```python
from build123d import *

# Parameters (mm, degrees)
F0_W     = 158.75
F0_H     = 6.35
F0_W_2   = 6.35
F0_H_2   = 95.25
F1_DEPTH = 19.05
F2_R     = 2.032
F3_DEPTH = 15.24
F4_R     = 2.032
F5_DEPTH = 25.4


with BuildPart() as f1:
    # F0 (on Top) → F1 (new body)
    with BuildSketch(Plane.XY):
        with Locations((-7.746776, 11.7905)):
            Rectangle(F0_W, F0_H)
        with Locations((74.803224, 11.7905)):
            Rectangle(F0_W_2, F0_H)
        with Locations((74.803224, -39.0095)):
            Rectangle(F0_W_2, F0_H_2)
    extrude(amount=F1_DEPTH)

    # F2 (on face) → F3 (cut)
    with BuildSketch(Plane.XZ.offset(86.6345)):
        with Locations((74.803224, 15.875)):
            Circle(F2_R)
        with Locations((74.803224, 3.175)):
            Circle(F2_R)
    extrude(amount=-F3_DEPTH, mode=Mode.SUBTRACT)

    # F4 (on face) → F5 (cut)
    with BuildSketch(Plane(origin=(0, 14.9655, 0), x_dir=(-1, 0, 0), z_dir=(0, 1, 0))):
        with Locations((83.946776, 15.875)):
            Circle(F4_R)
        with Locations((83.946776, 3.175)):
            Circle(F4_R)
    extrude(amount=-F5_DEPTH, mode=Mode.SUBTRACT)


solid = f1.part
```
Here's how the part is built. I have some questions about the finished solid (model axes, mm). A direction names the side the tool comes from. Round coordinates to 2 decimals unless told otherwise and drop trailing zeros. Write each loop counter-clockwise with the first axis right and the second up, starting at its lowest first coordinate (ties: lowest second). Pieces come first, ordered by that corner, then holes. Notation, with made-up numbers: M 49.5,28 L 60.5,28 A33 ccw 60.5,64 Z; hole C -26,30.25 d5. An arc over 180 degrees is marked long. Answer as CSV lines item,"result". Start each with the question number.
1. Suppose I cut it at D-D on y = -75.5. Write out the boundary of the cut face in (x, z) (3 decimals).
2. Thinking about a two-plate mould opening in X: for faces 4 (the flat face through (77.978, -37, 9)), 5 (the cylindrical face through (76.68, -79.12, 2.4)), 6 (the flat face through (75, -86.634, 9)), which applies, released by +X, released by -X, zero draft, split by the parting line, or undercut?
3. I need wall thicknesses on probe 1 along Y at (x, z) = (48, 7.25); probe 2 along X at (y, z) = (-64, 11). Which ranges of each line are inside material? Lowest first, please.
4. Suppose I cut it at B-B on y = -36.5. Write out the boundary of the cut face in (x, z).
5. On a 3-axis mill with a long thin cutter (end or side, diameter ignored), from which of +Z, -Z, +X, -X, +Y, -Y can I reach the whole of each face in a straight line? I mean faces 1 (the flat face through (71.628, -40, 9)), 2 (the flat face through (75, -71.395, 16)), 3 (the flat face through (-3, 14.965, 9)). Say none if no direction works.
6. Suppose I cut it at C-C on x = -27. Write out the boundary of the cut face in (y, z).
7. I'm going to push flat-ended pins straight in: pin 1 Ø5.5 at (x, z) = (7, 7.5) entering from -Y; pin 2 Ø9.5 at (y, z) = (-25.5, 10) entering from -X; pin 3 Ø3.5 at (x, z) = (-83.95, 3.18) entering from -Y; pin 4 Ø2 at (x, z) = (75, 4) entering from -Y. Where does each tip first touch, or does it pass through?
8. Suppose I cut it at A-A on z = 8.75. Write out the boundary of the cut face in (x, y).
Check result:
1,outline,"M 71.628,0 L 77.978,0 L 77.978,19.05 L 71.628,19.05 Z; hole C 74.803,3.175 d4.064; hole C 74.803,15.875 d4.064"
2,face 4,"released by +X"
2,face 5,"undercut"
2,face 6,"zero draft"
3,probe 1,"y = 8.62 to 14.97"
3,probe 2,"x = 71.63 to 77.98"
4,outline,"M 71.63,0 L 77.98,0 L 77.98,19.05 L 71.63,19.05 Z"
5,face 1,"+Z, -Z, -X, -Y"
5,face 2,"-Y"
5,face 3,"+Z, -Z, +X, -X, +Y"
6,outline,"M 8.62,0 L 14.97,0 L 14.97,19.05 L 8.62,19.05 Z"
7,pin 1,"stops at y = 8.62"
7,pin 2,"stops at x = 71.63"
7,pin 3,"passes through"
7,pin 4,"stops at y = -71.39"
8,outline,"M -87.12,8.62 L 71.63,8.62 L 71.63,-86.63 L 77.98,-86.63 L 77.98,14.97 L -87.12,14.97 Z"
